Autodesk Inventor part; units mm, degrees
ref_plane "YZ Plane" through (0, 0, 0) normal (1, 0, 0) x (0, 1, 0)
ref_plane "XZ Plane" through (0, 0, 0) normal (0, 1, 0) x (-1, 0, 0)
ref_plane "XY Plane" through (0, 0, 0) normal (0, 0, 1) x (1, 0, 0)
sketch "Skizze1" plane through (0, 0, 0) normal (0, 0, 1) x (1, 0, 0)
  line L0 (-21, 0) -> (21, 0)
  line L1 (0, -30.3276) -> (0, 25.6724)
  line L2 (-15, 17.6724) -> (15, 17.6724)
  line L3 (15, 17.6724) -> (15, -22.3276)
  line L4 (15, -22.3276) -> (-15, -22.3276)
  line L5 (-15, -22.3276) -> (-15, 17.6724)
  point P0 (0, 0)
  dimension "d0" = 40
  dimension "d1" = 30
extrude "Extrusion1" add sketch "Skizze1" along normal blind 20
sketch "Skizze5" plane through (0, 0, 20) normal (0, 0, 1) x (1, 0, 0)
  circle A0 centre (0, -2.3276) radius 2.5
  line L0 (15, 17.6724) -> (-15, 17.6724)
  point P0 (0, 0)
  dimension "d22" = 5
  dimension "d23" = 20
extrude "Extrusion5" add sketch "Skizze5" along normal blind 2
sketch "Skizze6" plane through (0, -2.3276, 22) normal (0, 0, 1) x (1, 0, 0)
  circle A0 centre (0, 0) radius 2.5
  line L0 (-2.5, 0) -> (2.5, 0)
  line L1 (1.7678, 1.7678) -> (0, 0)
  line L2 (0, 0) -> (-1.7678, -1.7678)
  line L3 (1.7678, 1.7678) -> (22.981, -19.4454)
  line L4 (22.981, -19.4454) -> (19.4454, -22.981)
  line L5 (19.4454, -22.981) -> (-1.7678, -1.7678)
  circle A1 centre (19.4454, -19.4454) radius 1.4773
  point P0 (0, 2.3276)
  dimension "d26" = 45
  dimension "d27" = 30
  dimension "d28" = 2.5
  dimension "d29" = 2.5
extrude "Extrusion6" add sketch "Skizze6" along normal blind 3
properties part number "Motor"
Geometry check sheet. Reference: the model listing, model coordinates, mm. A direction names the side the tool comes from. Coordinates: 2 decimals unless noted, no trailing zeros. Write each loop counter-clockwise with the first axis right and the second up, starting at its lowest first coordinate (ties: lowest second). Pieces come first, ordered by that corner, then holes. Notation, with made-up numbers: (16.25, 37.25) -> (57.25, 37.25) arc R37 cw to (57.25, 75.25) -> close; hole circle Ø2 at (-20, -9.5). An arc over 180 degrees is marked (long way). Use CSV: the item, a comma, the result in double quotes. Start each with the question number.
Item 1: Cross-section at A-A, the plane x = 4.5. Record the cut outline in (y, z), plus the area to 3 significant figures.
Item 2: Cross-section at B-B, the plane y = -19. Record the cut outline in (x, z).
Item 3: Thickness scan on line 1 (Z direction, x = 13.5, y = -16); line 2 (X direction, y = -21, z = 14.5); line 3 (Y direction, x = -12, z = 13.75). Record the ranges inside material, lowest first.
Item 4: Cross-section at C-C, the plane y = 12.5. Record the cut outline in (x, z).
Item 5: Set-up check for faces 1 (the flat face through (12.23, -11.02, 23.48)), 2 (the cylindrical face through (-1.984, -0.806, 21.909)), 3 (the flat face through (8.987, -14.85, 23.479)): record each of +Z, -Z, +X, -X, +Y, -Y from which the full face is reachable in a straight line by a thin tool's end or side.
Item 6: Depth check by flat-ended pin: pin 1 Ø2 at (y, z) = (9.5, 4) entering from +X; pin 2 Ø2.5 at (x, y) = (19.45, -21.77) entering from -Z; pin 3 Ø1.5 at (x, y) = (-9.5, -17.5) entering from +Z. Enter the tip coordinate at first touch or a pass-through.
Item 7: Mould release check, pull along Y, two halves, no side actions. Record for faces 4 (the flat face through (0, 17.672, 10)), 5 (the cylindrical face through (19.13, -20.33, 23.48)), 6 (the flat face through (0, -22.328, 10)): released by +Y, released by -Y, zero draft, split by the parting line, or undercut.
Item 8: Cross-section at D-D, the plane z = 17. Record the cut outline in (x, y).
Answers:
1,outline,"(-22.33, 0) -> (17.67, 0) -> (17.67, 20) -> (-22.33, 20) -> close; (-10.36, 22) -> (-3.29, 22) -> (-3.29, 25) -> (-10.36, 25) -> close"
1,area,"821 mm^2"
2,outline,"(-15, 0) -> (15, 0) -> (15, 20) -> (-15, 20) -> close; (13.14, 22) -> (20.21, 22) -> (20.21, 25) -> (13.14, 25) -> close"
3,line 1,"0 to 20, 22 to 25"
3,line 2,"-15 to 15"
3,line 3,"-22.33 to 17.67"
4,outline,"(-15, 0) -> (15, 0) -> (15, 20) -> (-15, 20) -> close"
5,face 1,"+Z, +X, +Y"
5,face 2,"none"
5,face 3,"+Z, -X, -Y"
6,pin 1,"x = 15"
6,pin 2,"through"
6,pin 3,"z = 20"
7,face 4,"released by +Y"
7,face 5,"undercut"
7,face 6,"released by -Y"
8,outline,"(-15, -22.33) -> (15, -22.33) -> (15, 17.67) -> (-15, 17.67) -> close"
